Geometry check sheet. Reference: the model listing, model coordinates, mm. Face numbers are marked on the shaded views. A direction names the side the tool comes from. Round coordinates to 2 decimals unless told otherwise and drop trailing zeros. Order: outer loops, then holes, each group sorted by start corner. A loop starts at its lowest first (then second) coordinate and runs counter-clockwise, first axis right, second up.
(1) Sectioned sample at D-D (x = 26). Record the boundary of the cut face in (y, z).
(2) Release check for a two-part mould opening along Y. For the marked faces 5, 6 and 7 record: +Y half, -Y half, draft (parallel to the pull), parting line (faces both ways), or undercut.
(3) Material ranges on line 1 along X through (y, z) = (7, -1.5); line 2 along Z through (x, y) = (15.5, -2.25); line 3 along Y through (x, z) = (2, 0), recorded low to high.
(4) Sectioned sample at C-C (y = -2.25). Give the number of separate pieces and of enclosed holes in the cut face, plus the area to 3 significant figures.
(5) Sectioned sample at B-B (z = 16). Record the boundary of the cut face in (x, y), plus the area to 3 significant figures.
(6) Set-up check for the marked faces 1, 2, 3 and 4: record each of +Z, -Z, +X, -X, +Y, -Y from which the full face is reachable in a straight line by a thin tool's end or side.
(7) Go/stop test with flat-tipped pins: pin 1 (1 mm diameter, centred on x = -2.5, y = -7, fed in from -Z); pin 2 (1.5 mm diameter, centred on x = 9.5, z = -3.5, fed in from -Y); pin 3 (4 mm diameter, centred on x = -8, y = 2, fed in from +Z); pin 4 (5.5 mm diameter, centred on y = -1.5, z = 1.5, fed in from +X) (3 decimals). Record where each tip stops, or that it passes through.
from build123d import *
from build123d.topology import SkipClean

# Parameters (mm, degrees)
SKETCH_2_R          = 8
SKETCH_2_R_2        = 4
EXTRUDE_1_DEPTH     = 26.1
SKETCH_4_R          = 8
EXTRUDE_2_DEPTH     = 13.05
SKETCH_6_R          = 5
CUT_EXTRUDE_1_DEPTH = 63.05
SKETCH_7_R          = 5
CUT_EXTRUDE_2_DEPTH = 25


with BuildPart() as part:
    # Эскиз1 → Повернуть1 (revolve)
    with BuildSketch(Plane.XY, mode=Mode.PRIVATE) as revolve_1_sk:
        Polygon((-16.75, -8), (-16.75, -6), (-15.75, -6), (-15.75, -8.75), (-15, -9.5), (-13.75, -9.5), (-13.75, -9), (-13, -9), (-13, -10), (-5, -10), (-5, -4), (-17.75, -4), (-17.75, -8), align=None)
    revolve(revolve_1_sk.sketch.rotate(Axis((-21.049489232, 0, 0), (1, 0, 0)), 270), axis=Axis((-21.049489232, 0, 0), (1, 0, 0)))

    # Эскиз2 → Бобышка-Вытянуть1 (add)
    with BuildSketch(Plane(origin=(-5, 0, 0), x_dir=(0, 0, -1), z_dir=(1, 0, 0))):
        with Locations(Location((0, 0, 0), (0, 0, 180))):
            Circle(SKETCH_2_R)
        with Locations(Location((0, 0, 0), (0, 0, 180))):
            Circle(SKETCH_2_R_2, mode=Mode.SUBTRACT)
    extrude(amount=EXTRUDE_1_DEPTH)

    # Эскиз3 → Повернуть2 (revolve)
    with SkipClean():  # the faces are left unmerged after this step: merging them gives an invalid solid
        with BuildSketch(Plane.XY):
            Polygon((32.85, 8), (32.85, 6), (31.85, 6), (31.85, 8.75), (31.1, 9.5), (29.85, 9.5), (29.85, 9), (29.1, 9), (29.1, 10), (21.1, 10), (21.1, 4), (33.85, 4), (33.85, 8), align=None)
        revolve(axis=Axis((47.149489232, 0, 0), (-1, 0, 0)))

    # Эскиз4 → Бобышка-Вытянуть2 (add)
    with SkipClean():  # the faces are left unmerged after this step: merging them gives an invalid solid
        with BuildSketch(Plane.XY):
            with Locations(Location((8.05, 0, 0), (0, 0, 90))):
                Circle(SKETCH_4_R)
        extrude(amount=EXTRUDE_2_DEPTH)

    # Эскиз5 → Повернуть3 (revolve)
    with SkipClean():  # the faces are left unmerged after this step: merging them gives an invalid solid
        with BuildSketch(Plane(origin=(0, 0, 0), x_dir=(1, 0, 0), z_dir=(0, 1, 0))):
            Polygon((16.05, -24.8), (14.05, -24.8), (14.05, -23.8), (16.8, -23.8), (17.55, -23.05), (17.55, -21.8), (17.05, -21.8), (17.05, -21.05), (18.05, -21.05), (18.05, -13.05), (12.05, -13.05), (12.05, -25.8), (16.05, -25.8), align=None)
        revolve(axis=Axis((8.05, 0, 29.099489232), (0, 0, -1)))

    # Эскиз6 → Вырез-Вытянуть1 (cut)
    with BuildSketch(Plane.ZY.offset(17.75)):
        Circle(SKETCH_6_R)
    extrude(amount=-CUT_EXTRUDE_1_DEPTH, mode=Mode.SUBTRACT)

    # Эскиз7 → Вырез-Вытянуть2 (cut)
    with BuildSketch(Plane.XY.offset(25.8)):
        with Locations((8.05, 0)):
            Circle(SKETCH_7_R)
    extrude(amount=-CUT_EXTRUDE_2_DEPTH, mode=Mode.SUBTRACT)


solid = part.part
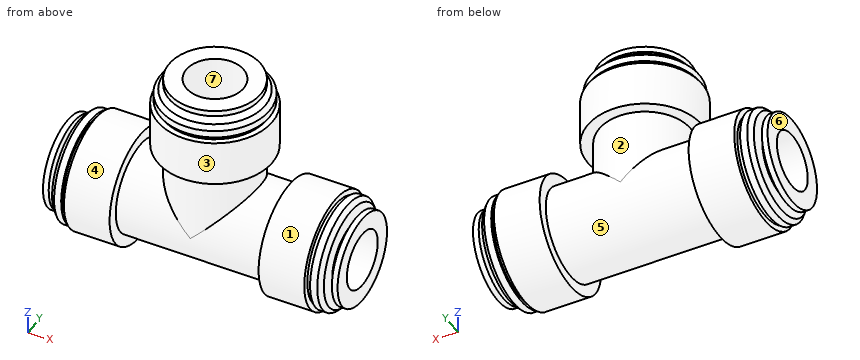
Answer below:
1. outline: circle Ø20 at (0, 0); hole circle Ø10 at (0, 0)
2. face 5: parting line
2. face 6: draft
2. face 7: undercut
3. line 1: x = -17.75 to -16.75, -15.75 to 31.85, 32.85 to 33.85
3. line 2: z = -7.68 to -4.47, 4.47 to 23.8, 24.8 to 25.8
3. line 3: y = -8 to -5, 5 to 8
4. separate pieces: 3
4. enclosed holes: 0
4. area: 527 mm2
5. outline: circle Ø20 at (8.05, 0); hole circle Ø10 at (8.05, 0)
5. area: 236 mm2
6. face 1: +X
6. face 2: none
6. face 3: +Z
6. face 4: -X
7. pin 1: stops at z = -4.66
7. pin 2: stops at y = -7.51
7. pin 3: stops at z = 10
7. pin 4: passes through
